Here's how the part is built. I have some questions about the finished solid (model axes, mm). Round coordinates to 2 decimals unless told otherwise and drop trailing zeros. Write each loop counter-clockwise with the first axis right and the second up, starting at its lowest first coordinate (ties: lowest second). Pieces come first, ordered by that corner, then holes. Notation, with made-up numbers: M 52.25,41 L 72.25,41 A12 ccw 72.25,60 Z; hole C -39,-7 d4. An arc over 180 degrees is marked long. Use one line per item in the form item = value. Start each with the question number.
Q1. I want a section at D-D on y = -19. List the corners of the cut face in (x, z) for me.
Q2. We'd pull the mould along X, two halves only. Please class faces 1 (the face through (-0.1, -4.2, 8)), 2 (the face through (-6.309, -28.413, 3.944)), 3 (the face through (-21.997, 0.631, 3.944)), 4 (the face through (-0.273, -5.918, 3.944)): +X half, -X half, draft (parallel to the pull), parting line (faces both ways), or undercut.
Q3. I'm going to push flat-ended pins straight in: pin 1 Ø4 at (x, y) = (-19, -11) entering from +Z; pin 2 Ø3 at (y, z) = (-11, 3.5) entering from -X; pin 3 Ø2.5 at (y, z) = (-12.5, 5.5) entering from -X; pin 4 Ø4 at (y, z) = (16, 5) entering from -X. Where does each tip first touch, or does it pass through?
Q4. I want a section at A-A on x = 0. State how many separate pieces and enclosed holes the cut face has, and give its area (3 significant figures).
Q5. I need wall thicknesses on line 1 along Y through (x, z) = (-8, 4); line 2 along X through (y, z) = (-6.5, 5.5); line 3 along Y through (x, z) = (-9.5, 1.25). Which ranges of each line are inside material? Lowest first, please. Write a range as from..to.
```python
from build123d import *

# Parameters (mm, degrees)
CROQUIS1_R              = 29.105
CROQUIS1_R_2            = 4
CROQUIS1_R_3            = 2.1
SALIENTE_EXTRUIR1_DEPTH = 8


with BuildPart() as part:
    # Croquis1 → Saliente-Extruir1 (new body)
    with BuildSketch(Plane.XY):
        Circle(CROQUIS1_R)
        Circle(CROQUIS1_R_2, mode=Mode.SUBTRACT)
        with BuildLine():
            ThreePointArc((6.6, 4), (3.771572875, 5.171572875), (2.6, 8))
            Line((2.6, 8), (2.6, 24.864432429))
            ThreePointArc((2.6, 24.864432429), (15.442895729, 19.66003488), (23.541098272, 8.415265423))
            ThreePointArc((23.541098272, 8.415265423), (22.942587119, 5.373198291), (20.162890285, 4))
            Line((20.162890285, 4), (6.6, 4))
        make_face(mode=Mode.SUBTRACT)
        with Locations((0, 24)):
            Circle(CROQUIS1_R_3, mode=Mode.SUBTRACT)
        with BuildLine():
            ThreePointArc((-8.415265423, 23.541098272), (-5.373198291, 22.942587119), (-4, 20.162890285))
            Line((-4, 20.162890285), (-4, 6.6))
            ThreePointArc((-4, 6.6), (-5.171572875, 3.771572875), (-8, 2.6))
            Line((-8, 2.6), (-24.864432429, 2.6))
            ThreePointArc((-24.864432429, 2.6), (-19.66003488, 15.442895729), (-8.415265423, 23.541098272))
        make_face(mode=Mode.SUBTRACT)
        with Locations((-24, 0)):
            Circle(CROQUIS1_R_3, mode=Mode.SUBTRACT)
        with BuildLine():
            ThreePointArc((-23.541098272, -8.415265423), (-22.942587119, -5.373198291), (-20.162890285, -4))
            Line((-20.162890285, -4), (-6.6, -4))
            ThreePointArc((-6.6, -4), (-3.771572875, -5.171572875), (-2.6, -8))
            Line((-2.6, -8), (-2.6, -24.864432429))
            ThreePointArc((-2.6, -24.864432429), (-15.442895729, -19.66003488), (-23.541098272, -8.415265423))
        make_face(mode=Mode.SUBTRACT)
        with Locations((0, -24)):
            Circle(CROQUIS1_R_3, mode=Mode.SUBTRACT)
        with BuildLine():
            ThreePointArc((8.415265423, -23.541098272), (5.373198291, -22.942587119), (4, -20.162890285))
            Line((4, -20.162890285), (4, -6.6))
            ThreePointArc((4, -6.6), (5.171572875, -3.771572875), (8, -2.6))
            Line((8, -2.6), (24.864432429, -2.6))
            ThreePointArc((24.864432429, -2.6), (19.66003488, -15.442895729), (8.415265423, -23.541098272))
        make_face(mode=Mode.SUBTRACT)
        with Locations((24, 0)):
            Circle(CROQUIS1_R_3, mode=Mode.SUBTRACT)
        with Locations((0, -8)):
            Circle(CROQUIS1_R_3, mode=Mode.SUBTRACT)
        with Locations((0, -16)):
            Circle(CROQUIS1_R_3, mode=Mode.SUBTRACT)
        with Locations((-8, 0)):
            Circle(CROQUIS1_R_3, mode=Mode.SUBTRACT)
        with Locations((-16, 0)):
            Circle(CROQUIS1_R_3, mode=Mode.SUBTRACT)
        with Locations((0, 8)):
            Circle(CROQUIS1_R_3, mode=Mode.SUBTRACT)
        with Locations((0, 16)):
            Circle(CROQUIS1_R_3, mode=Mode.SUBTRACT)
        with Locations((16, 0)):
            Circle(CROQUIS1_R_3, mode=Mode.SUBTRACT)
        with Locations((8, 0)):
            Circle(CROQUIS1_R_3, mode=Mode.SUBTRACT)
    extrude(amount=SALIENTE_EXTRUIR1_DEPTH)


solid = part.part
```
Reported:
q1.outline = M -22.05,0 L -16.25,0 L -16.25,8 L -22.05,8 Z; M -2.6,0 L 4,0 L 4,8 L -2.6,8 Z; M 16.25,0 L 22.05,0 L 22.05,8 L 16.25,8 Z
q2.face_1 = draft
q2.face_2 = parting line
q2.face_3 = undercut
q2.face_4 = undercut
q3.pin_1 = through
q3.pin_2 = -27.51
q3.pin_3 = -26.84
q3.pin_4 = -25.52
q4.separate_pieces = 8
q4.enclosed_holes = 0
q4.area = 200 mm^2
q5.line_1 = -27.98..-23.69, -4..-2.1, 2.1..2.6, 23.63..27.98
q5.line_2 = -28.37..-23.52, -2.89..-1.47, 1.47..4, 24.14..28.37
q5.line_3 = -27.51..-23.12, -4..-1.47, 1.47..2.6, 23.12..27.51
